The drawing under review shows one solid part. Ordinate dimensions are in mm from its lowest x, y, z. Give positions to 0.01 mm unless a question says otherwise; leave off trailing zeros. Loops run counter-clockwise (first coordinate to the right, second up) from the corner with the lowest first, then second, coordinate; pieces in that order, holes last. Notation, with made-up numbers: (9.25, 30.5) -> (26.25, 30.5) arc R12 ccw to (26.25, 45.5) -> close; hole circle Ø9 at (46.5, 50). An arc over 180 degrees is marked (long way). Answer in a Markdown table with one row per item. Add a question column.
(1) For line 1 (Y direction, x = 8.25, z = 20); line 2 (Y direction, x = 8.5, z = 14.5), list the stretches that pass through material, from the lowest coordinate up.
(2) Consider section A-A on x = 5.5. Write out the cut boundary in (y, z).
(3) For pin 1 (1.5 mm diameter, centred on y = 87, z = 35, fed in from -X); pin 2 (3 mm diameter, centred on x = 9, z = 4.5, fed in from +Y); pin 3 (9.5 mm diameter, centred on y = 12.5, z = 20, fed in from +X), all flat-tipped, find the tip position at first contact; note any pin that passes through.
(4) Consider section C-C on z = 21. Write out the cut boundary in (x, y), then the cut area to 3 significant figures.
(5) Consider section B-B on y = 222.5. Write out the cut boundary in (x, z), then the cut area to 3 significant figures.
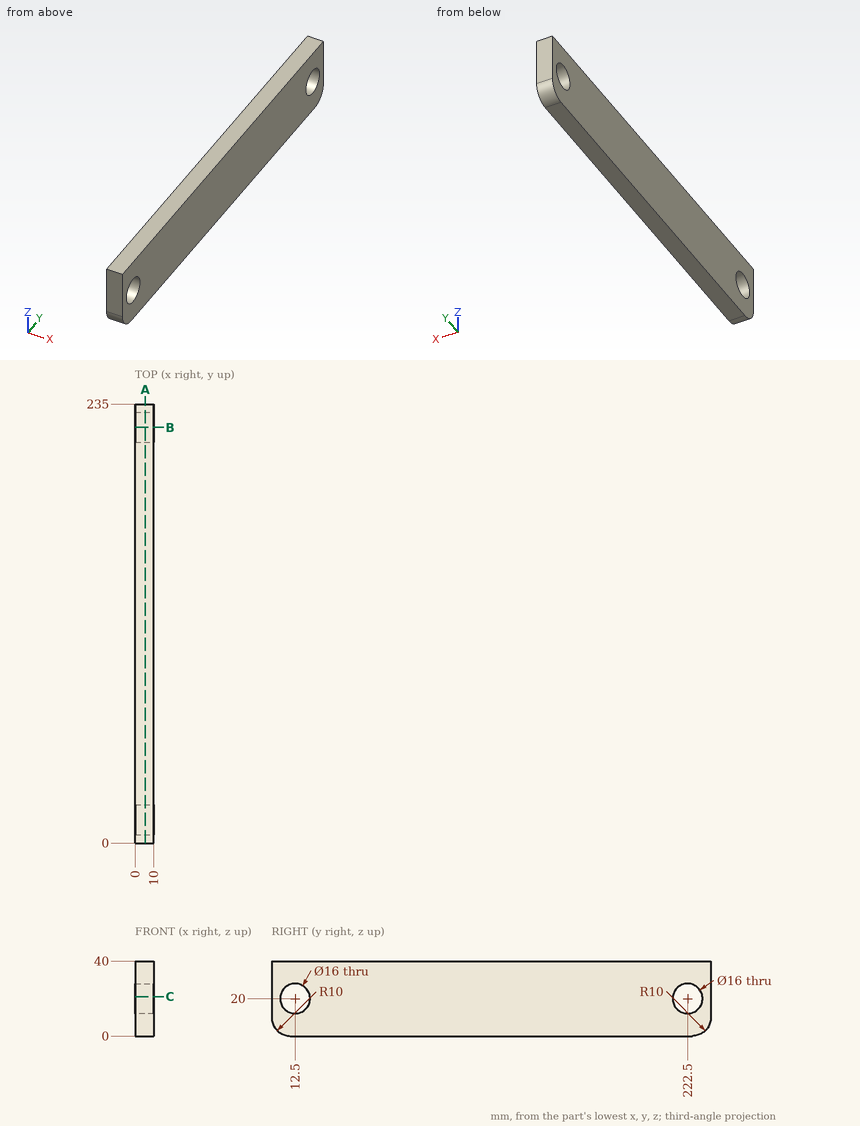
Values follow:
| question | item | result |
|---|---|---|
| 1 | line 1 | 0 to 4.5, 20.5 to 214.5, 230.5 to 235 |
| 1 | line 2 | 0 to 6.69, 18.31 to 216.69, 228.31 to 235 |
| 2 | outline | (0, 10) arc R10 ccw to (10, 0) -> (225, 0) arc R10 ccw to (235, 10) -> (235, 40) -> (0, 40) -> close; hole circle Ø16 at (12.5, 20); hole circle Ø16 at (222.5, 20) |
| 3 | pin 1 | x = 0 |
| 3 | pin 2 | y = 234.17 |
| 3 | pin 3 | through |
| 4 | outline | (0, 0) -> (10, 0) -> (10, 4.56) -> (0, 4.56) -> close; (0, 20.44) -> (10, 20.44) -> (10, 214.56) -> (0, 214.56) -> close; (0, 230.44) -> (10, 230.44) -> (10, 235) -> (0, 235) -> close |
| 4 | area | 2,030 mm2 |
| 5 | outline | (0, 0) -> (10, 0) -> (10, 12) -> (0, 12) -> close; (0, 28) -> (10, 28) -> (10, 40) -> (0, 40) -> close |
| 5 | area | 240 mm2 |
